Read the model definition and answer for the solid it produces. Units are mm, in the model's axes. A direction names the side the tool comes from. Round coordinates to 2 decimals unless told otherwise and drop trailing zeros. Write each loop counter-clockwise with the first axis right and the second up, starting at its lowest first coordinate (ties: lowest second). Pieces come first, ordered by that corner, then holes. Notation, with made-up numbers: (36.25, 49) -> (40.25, 49) arc R18 cw to (40.25, 58) -> close; hole circle Ø11 at (4, 64.5). An arc over 180 degrees is marked (long way). Return JSON: item names as keys, results as strings.
from build123d import *

# Parameters (mm, degrees)
SKETCH_1_W                = 22
SKETCH_1_H                = 13
EXTRUDE_1_DEPTH           = 33
SKETCH_5_W                = 30
SKETCH_5_H                = 13
CUT_EXTRUDE_2_DEPTH       = 17
HOLE_WIZARD_1_D           = 3.4
HOLE_WIZARD_1_CBORE_D     = 6
HOLE_WIZARD_1_CBORE_DEPTH = 3
CUT_EXTRUDE_4_DEPTH       = 36.387144558
FILLET_1_R                = 3


with BuildPart() as part:
    # 草图1 → 凸台-拉伸1 (new body)
    with BuildSketch(Plane.XY):
        Rectangle(SKETCH_1_W, SKETCH_1_H)
    extrude(amount=EXTRUDE_1_DEPTH)

    # 草图5 → 切除-拉伸2 (cut)
    with BuildSketch(Plane.ZY.offset(11)):
        with Locations((15, 0)):
            Rectangle(SKETCH_5_W, SKETCH_5_H)
    extrude(amount=-CUT_EXTRUDE_2_DEPTH, mode=Mode.SUBTRACT)

    # 打孔尺寸根据内六角圆柱头螺钉的类型1 (through all)
    with Locations(Plane(origin=(6, 5.532872615, -4.059557146), x_dir=(0, 0, 1), z_dir=(-1, 0, 0))):
        with Locations((28.059557146, -8.532872615), (8.059557146, -8.532872615)):
            CounterBoreHole(HOLE_WIZARD_1_D / 2, HOLE_WIZARD_1_CBORE_D / 2, HOLE_WIZARD_1_CBORE_DEPTH)

    # 草图12 → 切除-拉伸4 (cut, through all)
    with BuildSketch(Plane.XY.offset(33)):
        with BuildLine():
            Line((-11, -3.5), (-6, -3.5))
            ThreePointArc((-6, -3.5), (-2.5, 0), (-6, 3.5))
            Line((-6, 3.5), (-11, 3.5))
            Line((-11, 3.5), (-11, -3.5))
        make_face()
    extrude(amount=-CUT_EXTRUDE_4_DEPTH, mode=Mode.SUBTRACT)

    # 圆角1
    fillet_1_edges = [part.edges().sort_by_distance(p)[0] for p in [
        (6, 0, 30),
    ]]
    fillet(fillet_1_edges, radius=FILLET_1_R - 0.0001)  # a hair under: the kernel refuses the full size


solid = part.part
Item 1: Section A-A (z = 4) is taken. Give the vertices of the cut face in (x, y), then the cut area to 3 significant figures.
Worked answers:
{"outline": "(6, -6.5) -> (11, -6.5) -> (11, -4.7) -> (9, -4.7) -> (9, -6) -> (6, -6) -> close; (6, 0) -> (9, 0) -> (9, -1.3) -> (11, -1.3) -> (11, 6.5) -> (6, 6.5) -> close", "area": "40.2 mm2"}
Item 2: Section B-B (x = -7) is taken. Give the vertices of the cut face in (y, z).
Worked answers:
{"outline": "(-6.5, 30) -> (-3.5, 30) -> (-3.5, 33) -> (-6.5, 33) -> close; (3.5, 30) -> (6.5, 30) -> (6.5, 33) -> (3.5, 33) -> close"}
Item 3: Straight lines are drawn through the part: L1, parallel to Y at x = 9.5, z = 24; L2, parallel to Y at x = -8.5, z = 32; L3, parallel to X at y = 1, z = 14. For each, find the intervals that lie inside material, in ascending order. Write a range as [from, to].
Worked answers:
{"L1": "y = [-6.5, -4.7], [-1.3, 6.5]", "L2": "y = [-6.5, -3.5], [3.5, 6.5]", "L3": "x = [6, 11]"}
Item 4: Flat-ended cylindrical pins translate along their axes: pin 1 (6.5 mm diameter, centred on y = -1.5, z = 4.5, fed in from -X); pin 2 (4 mm diameter, centred on x = -4, y = 3, fed in from -Z); pin 3 (3 mm diameter, centred on y = -3, z = 4, fed in from +X). Find the tip coordinate at first contact, or state that the pin passes through.
Worked answers:
{"pin 1": "stops at x = 6", "pin 2": "stops at z = 30", "pin 3": "passes through"}
Item 5: For a pull along Z with two mould halves and no side action, classify faces 1 (the cylindrical face through (7, -3, 21)), 2 (the cylindrical face through (-2.5, -0.1, 31.5)), 3 (the cylindrical face through (5.1, 0.09, 29.14)) as released by +Z, released by -Z, zero draft, split by the parting line, or undercut.
Worked answers:
{"face 1": "undercut", "face 2": "zero draft", "face 3": "released by -Z"}
Item 6: Section D-D (y = 5.25) is taken. Give the vertices of the cut face in (x, z), then the cut area to 3 significant figures.
Worked answers:
{"outline": "(-11, 30) -> (3, 30) arc R3 cw to (6, 27) -> (6, 0) -> (11, 0) -> (11, 33) -> (-11, 33) -> close", "area": "218 mm2"}
Item 7: A tool of negligible diameter and unlimited length cuts with its end or side. For faces 4 (the flat face through (9, -5, 4)), 5 (the flat face through (2, 0, 33)), 6 (the flat face through (-2.5, -1.5, 30)), 7 (the flat face through (-9, -3.5, 32)), from which of +Z, -Z, +X, -X, +Y, -Y can it reach the whole face along a straight path? Write none if from no direction.
Worked answers:
{"face 4": "-X", "face 5": "+Z, +X, -X, +Y, -Y", "face 6": "-Z, -X, +Y, -Y", "face 7": "+Z, -Z, -X"}
Item 8: Section C-C (y = -3) is taken. State how many separate pieces and enclosed holes the cut face has, then the cut area to 3 significant figures.
Worked answers:
{"separate pieces": "3", "enclosed holes": "0", "area": "148 mm2"}
